Read the model definition and answer for the solid it produces. Units are mm, in the model's axes. Face numbers are marked on the shaded views. A direction names the side the tool comes from. Coordinates: 2 decimals unless noted, no trailing zeros. Loops run counter-clockwise (first coordinate to the right, second up) from the corner with the lowest first, then second, coordinate; pieces in that order, holes last.
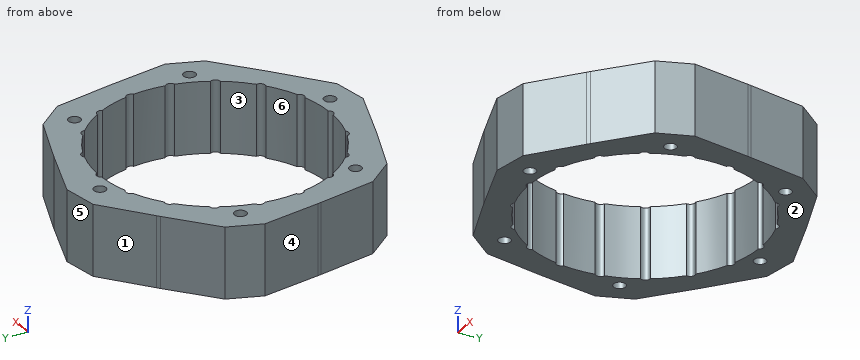
from build123d import *

# Parameters (mm, degrees)
SKETCH1_R           = 60
BOSS_EXTRUDE1_DEPTH = 30
SKETCH2_R           = 2.55
CUT_EXTRUDE2_DEPTH  = 91
BOSS_EXTRUDE2_START = -30
BOSS_EXTRUDE2_DEPTH = 30


with BuildPart() as part:
    # Sketch1 → Boss-Extrude1 (new body)
    with BuildSketch(Plane.XY):
        Circle(SKETCH1_R)
        with BuildLine():
            ThreePointArc((-15.015830627, 46.642521701), (-17.128368778, 47.059806449), (-18.478441423, 45.382234438))
            ThreePointArc((-18.478441423, 45.382234438), (-24.5, 42.435244785), (-30.062947192, 38.693916914))
            ThreePointArc((-30.062947192, 38.693916914), (-32.190803493, 38.363505711), (-32.885693376, 36.325351632))
            ThreePointArc((-32.885693376, 36.325351632), (-37.536177713, 31.496592875), (-41.484028644, 26.078254686))
            ThreePointArc((-41.484028644, 26.078254686), (-43.370552222, 25.04), (-43.326445366, 22.887095314))
            ThreePointArc((-43.326445366, 22.887095314), (-46.044938419, 16.758987023), (-47.901524003, 10.317170068))
            ThreePointArc((-47.901524003, 10.317170068), (-49.319172271, 8.696300738), (-48.541388615, 6.688317524))
            ThreePointArc((-48.541388615, 6.688317524), (-49, 0), (-48.541388615, -6.688317524))
            ThreePointArc((-48.541388615, -6.688317524), (-49.319172271, -8.696300738), (-47.901524003, -10.317170068))
            ThreePointArc((-47.901524003, -10.317170068), (-46.044938419, -16.758987023), (-43.326445366, -22.887095314))
            ThreePointArc((-43.326445366, -22.887095314), (-43.370552222, -25.04), (-41.484028644, -26.078254686))
            ThreePointArc((-41.484028644, -26.078254686), (-37.536177713, -31.496592875), (-32.885693376, -36.325351632))
            ThreePointArc((-32.885693376, -36.325351632), (-32.190803493, -38.363505711), (-30.062947192, -38.693916914))
            ThreePointArc((-30.062947192, -38.693916914), (-24.5, -42.435244785), (-18.478441423, -45.382234438))
            ThreePointArc((-18.478441423, -45.382234438), (-17.128368778, -47.059806449), (-15.015830627, -46.642521701))
            ThreePointArc((-15.015830627, -46.642521701), (-8.508760706, -48.255579898), (-1.842416722, -48.96535))
            ThreePointArc((-1.842416722, -48.96535), (0, -50.08), (1.842416722, -48.96535))
            ThreePointArc((1.842416722, -48.96535), (8.508760706, -48.255579898), (15.015830627, -46.642521701))
            ThreePointArc((15.015830627, -46.642521701), (17.128368778, -47.059806449), (18.478441423, -45.382234438))
            ThreePointArc((18.478441423, -45.382234438), (24.5, -42.435244785), (30.062947192, -38.693916914))
            ThreePointArc((30.062947192, -38.693916914), (32.190803493, -38.363505711), (32.885693376, -36.325351632))
            ThreePointArc((32.885693376, -36.325351632), (37.536177713, -31.496592875), (41.484028644, -26.078254686))
            ThreePointArc((41.484028644, -26.078254686), (43.370552222, -25.04), (43.326445366, -22.887095314))
            ThreePointArc((43.326445366, -22.887095314), (46.044938419, -16.758987023), (47.901524003, -10.317170068))
            ThreePointArc((47.901524003, -10.317170068), (49.319172271, -8.696300738), (48.541388615, -6.688317524))
            ThreePointArc((48.541388615, -6.688317524), (49, 0), (48.541388615, 6.688317524))
            ThreePointArc((48.541388615, 6.688317524), (49.319172271, 8.696300738), (47.901524003, 10.317170068))
            ThreePointArc((47.901524003, 10.317170068), (46.044938419, 16.758987023), (43.326445366, 22.887095314))
            ThreePointArc((43.326445366, 22.887095314), (43.370552222, 25.04), (41.484028644, 26.078254686))
            ThreePointArc((41.484028644, 26.078254686), (37.536177713, 31.496592875), (32.885693376, 36.325351632))
            ThreePointArc((32.885693376, 36.325351632), (32.190803493, 38.363505711), (30.062947192, 38.693916914))
            ThreePointArc((30.062947192, 38.693916914), (24.5, 42.435244785), (18.478441423, 45.382234438))
            ThreePointArc((18.478441423, 45.382234438), (17.128368778, 47.059806449), (15.015830627, 46.642521701))
            ThreePointArc((15.015830627, 46.642521701), (8.508760706, 48.255579898), (1.842416722, 48.96535))
            ThreePointArc((1.842416722, 48.96535), (0, 50.08), (-1.842416722, 48.96535))
            ThreePointArc((-1.842416722, 48.96535), (-8.508760706, 48.255579898), (-15.015830627, 46.642521701))
        make_face(mode=Mode.SUBTRACT)
    extrude(amount=BOSS_EXTRUDE1_DEPTH)

    # Sketch2 → Cut-Extrude2 (cut, through all)
    with BuildSketch(Plane.XY.offset(30)):
        with Locations((-9.550649772, 54.164426416)):
            Circle(SKETCH2_R)
        with Locations((42.132444372, 35.353318533)):
            Circle(SKETCH2_R)
        with Locations((51.683094143, -18.811107883)):
            Circle(SKETCH2_R)
        with Locations((9.550649772, -54.164426416)):
            Circle(SKETCH2_R)
        with Locations((-42.132444372, -35.353318533)):
            Circle(SKETCH2_R)
        with Locations((-51.683094143, 18.811107883)):
            Circle(SKETCH2_R)
    extrude(amount=-CUT_EXTRUDE2_DEPTH, mode=Mode.SUBTRACT)

    # Sketch3 → Boss-Extrude2 (add)
    with BuildSketch(Plane.XY.offset(30).offset(BOSS_EXTRUDE2_START)):
        with BuildLine():
            Line((-37.958811886, 46.46642444), (-18.597801703, 62.282596059))
            Line((-18.597801703, 62.282596059), (-3.825685408, 64.887318724))
            Line((-3.825685408, 64.887318724), (19.777162276, 56.646834442))
            ThreePointArc((19.777162276, 56.646834442), (-10.41889066, 59.088465181), (-37.958811886, 46.46642444))
        make_face()
        with BuildLine():
            Line((54.281223694, 35.756800112), (58.946178809, 11.195892275))
            ThreePointArc((58.946178809, 11.195892275), (45.962666587, 38.567256581), (21.261698045, 56.106507611))
            Line((21.261698045, 56.106507611), (44.639409549, 47.247466759))
            Line((44.639409549, 47.247466759), (54.281223694, 35.756800112))
        make_face()
        with BuildLine():
            Line((58.106909102, -29.130518612), (39.169016532, -45.450942167))
            ThreePointArc((39.169016532, -45.450942167), (56.381557247, -20.5212086), (59.220509931, 9.640083171))
            Line((59.220509931, 9.640083171), (63.237211252, -15.0351293))
            Line((63.237211252, -15.0351293), (58.106909102, -29.130518612))
        make_face()
        with BuildLine():
            Line((3.825685408, -64.887318724), (-19.777162276, -56.646834442))
            ThreePointArc((-19.777162276, -56.646834442), (10.41889066, -59.088465181), (37.958811886, -46.46642444))
            Line((37.958811886, -46.46642444), (18.597801703, -62.282596059))
            Line((18.597801703, -62.282596059), (3.825685408, -64.887318724))
        make_face()
        with BuildLine():
            Line((-54.281223694, -35.756800112), (-58.946178809, -11.195892275))
            ThreePointArc((-58.946178809, -11.195892275), (-45.962666587, -38.567256581), (-21.261698045, -56.106507611))
            Line((-21.261698045, -56.106507611), (-44.639409549, -47.247466759))
            Line((-44.639409549, -47.247466759), (-54.281223694, -35.756800112))
        make_face()
        with BuildLine():
            Line((-58.106909102, 29.130518612), (-39.169016532, 45.450942167))
            ThreePointArc((-39.169016532, 45.450942167), (-56.381557247, 20.5212086), (-59.220509931, -9.640083171))
            Line((-59.220509931, -9.640083171), (-63.237211252, 15.0351293))
            Line((-63.237211252, 15.0351293), (-58.106909102, 29.130518612))
        make_face()
    extrude(amount=BOSS_EXTRUDE2_DEPTH)


solid = part.part
Item 1: A cutting plane is placed at A-A on y = 42.5. Determine the outline of the cut face in (x, z), then the cut area to 3 significant figures.
Numbers:
outline: (-42.59, 0) - (-24.39, 0) - (-24.39, 30) - (-42.59, 30) - close; (24.39, 0) - (48.62, 0) - (48.62, 30) - (24.39, 30) - close
area: 1,270 mm2
Item 2: Find the intervals of material crossed by line 1 along X through (y, z) = (20, 16); line 2 along X through (y, z) = (-34, 14.5); line 3 along Y through (x, z) = (-44, 9.5), in increasing order.
Numbers:
line 1: x = -61.43 to -53.94, -49.43 to -44.73, 44.73 to 57.27
line 2: x = -54.61 to -44.29, -39.97 to -35.28, 35.28 to 52.46
line 3: y = -47.49 to -37.09, -33.62 to -21.56, 21.56 to 41.29
Item 3: Determine the mould class of the marked faces 1, 2, 3 and 4 for opening direction Y: released by +Y, released by -Y, zero draft, split by the parting line, or undercut.
Numbers:
face 1: released by +Y
face 2: zero draft
face 3: undercut
face 4: released by -Y
Item 4: A cutting plane is placed at B-B on x = -35.5. Determine the outline of the cut face in (y, z) (3 decimals).
Numbers:
outline: (-50.711, 0) - (-33.775, 0) - (-33.775, 30) - (-50.711, 30) - close; (33.775, 0) - (48.475, 0) - (48.475, 30) - (33.775, 30) - close
Item 5: Given pin 1 (2 mm diameter, centred on x = 47.5, z = 8.5, fed in from -Y); pin 2 (4.5 mm diameter, centred on x = -42.13, y = -35.35, fed in from +Z); pin 3 (8 mm diameter, centred on y = -13.5, z = 26.5, fed in from -X); pin 4 (1 mm diameter, centred on x = -39, z = 18, fed in from +Y), each flat-ended and moving along its own axis, determine where each tip first touches the part or whether it passes through.
Numbers:
pin 1: stops at y = -39.13
pin 2: passes through
pin 3: stops at x = -59.24
pin 4: stops at y = 46.02
Item 6: A cutting plane is placed at C-C on z = 27. Give the number of separate pieces and of enclosed holes in the cut face, then the cut area to 3 significant figures.
Numbers:
separate pieces: 1
enclosed holes: 7
area: 4,470 mm2
Item 7: Which of the six approach directions +Z, -Z, +X, -X, +Y, -Y give full straight-line access (tool end or side, diameter ignored) to the marked faces 5 and 6?
Numbers:
face 5: +Z, -Z, -X, +Y
face 6: +Z, -Z
